```python
from build123d import *

# Parameters (mm, degrees)
SKETCH1_R                 = 11.0998
SKETCH1_R_2               = 9.525
BOSS_EXTRUDE1_DEPTH       = 3.175
F_8_CLEARANCE_HOLE1_D     = 4.4958
F_8_CLEARANCE_HOLE1_DEPTH = 12.7
F_8_CLEARANCE_HOLE1_TIP   = 1.350674586
F_8_CLEARANCE_HOLE2_D     = 4.4958


with BuildPart() as part:
    # Sketch1 → Boss-Extrude1 (new body)
    with BuildSketch(Plane.XY):
        with BuildLine():
            Line((-188.264639147, 81.011774484), (56.809800323, 298.704514086))
            ThreePointArc((56.809800323, 298.704514086), (76.096805757, 305.388436009), (94.461024604, 296.476710194))
            Line((94.461024604, 296.476710194), (260.194034881, 109.897568099))
            ThreePointArc((260.194034881, 109.897568099), (271.059668812, 38.975929697), (210.82, 0))
            Line((210.82, 0), (-157.48, 0))
            ThreePointArc((-157.48, 0), (-200.811863601, 29.88880366), (-188.264639147, 81.011774484))
        make_face()
        with Locations((-157.48, 46.355)):
            Circle(SKETCH1_R, mode=Mode.SUBTRACT)
        with Locations((74.521510517, 278.765)):
            Circle(SKETCH1_R, mode=Mode.SUBTRACT)
        with Locations((210.82, 66.04)):
            Circle(SKETCH1_R, mode=Mode.SUBTRACT)
        with Locations((18.5166, 46.355)):
            Circle(SKETCH1_R_2, mode=Mode.SUBTRACT)
    extrude(amount=BOSS_EXTRUDE1_DEPTH)

    # #8 Clearance Hole1
    with Locations(Plane.XY.offset(3.175)):
        with Locations((36.477112242, 64.315512242), (36.477112242, 28.394487758), (0.556087758, 28.394487758), (0.556087758, 64.315512242)):
            Hole(F_8_CLEARANCE_HOLE1_D / 2, depth=F_8_CLEARANCE_HOLE1_DEPTH)
            with Locations((0, 0, -(F_8_CLEARANCE_HOLE1_DEPTH + F_8_CLEARANCE_HOLE1_TIP / 2))):  # 118° drill point
                Cone(0, F_8_CLEARANCE_HOLE1_D / 2, F_8_CLEARANCE_HOLE1_TIP, mode=Mode.SUBTRACT)

    # #8 Clearance Hole2 (through all)
    with Locations(Plane.XY.offset(3.175)):
        with Locations((17.768914495, 247.038768822), (36.758927911, 263.907064244), (110.26846103, 259.557542359), (127.136756453, 240.567528943), (208.528289616, 148.938453927), (225.396585039, 129.948440511), (270.394698688, 62.514995218), (253.027203769, 23.832796231), (172.72, 12.7), (147.32, 12.7), (-93.98, 12.7), (-119.38, 12.7), (-194.875991874, 32.144446994), (-151.345471312, 96.81921091), (-132.355457896, 113.687506333), (-55.88, 149.225), (-55.88, 92.075), (134.62, 92.075), (134.62, 149.225), (83.82, 200.025), (39.37, 120.65)):
            Hole(F_8_CLEARANCE_HOLE2_D / 2)


solid = part.part
```
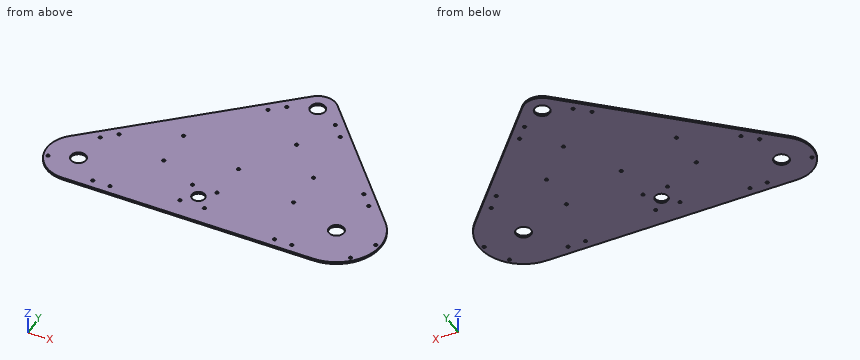
Source: CAD feature listing. Evaluate the final solid. Frame: model axes, mm. Coordinates: 2 decimals unless noted, no trailing zeros. Loops run counter-clockwise (first coordinate to the right, second up) from the corner with the lowest first, then second, coordinate; pieces in that order, holes last. Notation, with made-up numbers: M 63,32.5 L 120,32.5 A19 cw 120,40.5 Z; hole C -29,5.5 d4. An arc over 180 degrees is marked long. Use CSV: the item, a comma, the result in double quotes.
(1) Contact query for flat-ended pins moving along their axis: pin 1 (1 mm diameter, centred on x = 228, z = 2, fed in from +Y); pin 2 (8 mm diameter, centred on x = 29, y = 132, fed in from -Z); pin 3 (3.5 mm diameter, centred on x = 39.37, y = 120.65, fed in from +Z); pin 4 (1.5 mm diameter, centred on y = 256, z = 1, fed in from +X). Output: stop coordinate, or through.
Answers follow:
pin 1,"y = 146.7"
pin 2,"z = 0"
pin 3,"through"
pin 4,"x = 131.08"
(2) Cut plane A-A on y = 164. Return loops of the section in (x, z) (3 decimals), and give its area (3 significant figures).
Answers follow:
outline,"M -94.838,0 L 212.136,0 L 212.136,3.175 L -94.838,3.175 Z"
area,"975 mm²"
(3) Cut plane B-B on z = 1.4. Give the number of separate pieces and of enclosed holes in the cut face, and give its area (3 significant figures).
Answers follow:
separate pieces,"1"
enclosed holes,"29"
area,"91,100 mm²"
(4) Line query: line 1 (Y direction, x = 134.62, z = 0.85); line 2 (X direction, y = 128, z = 1.1); line 3 (X direction, y = 240, z = 0.3). Output: solid intervals per line, ascending. Write a range as [from, to].
Answers follow:
line 1,"[0, 89.83], [94.32, 146.98], [151.47, 251.27]"
line 2,"[-135.37, 224.28], [226.52, 244.11]"
line 3,"[-9.28, 124.96], [129.31, 144.63]"
(5) Cut plane C-C on x = 155.5. Return loops of the section in (y, z) (3 decimals), and give its area (3 significant figures).
Answers follow:
outline,"M 0,0 L 227.76,0 L 227.76,3.175 L 0,3.175 Z"
area,"723 mm²"
